```python
from build123d import *

# Parameters (mm, degrees)
BOSS_EXTRUDE1_DEPTH = 12.7
SKETCH2_R           = 2.286
SKETCH2_R_2         = 0.6
CUT_EXTRUDE1_DEPTH  = 3.175
FILLET1_R           = 2.54


with BuildPart() as part:
    # Sketch1 → Boss-Extrude1 (new body)
    with BuildSketch(Plane.XY):
        with BuildLine():
            Line((0, 26.364540169), (0, -11.735459831))
            ThreePointArc((0, -11.735459831), (0.371974388, -12.633485443), (1.27, -13.005459831))
            Line((1.27, -13.005459831), (13.97, -13.005459831))
            Line((13.97, -13.005459831), (13.97, -16.180459831))
            Line((13.97, -16.180459831), (1.27, -16.180459831))
            ThreePointArc((1.27, -16.180459831), (-1.873089642, -14.878549473), (-3.175, -11.735459831))
            Line((-3.175, -11.735459831), (-3.175, 26.364540169))
            Line((-3.175, 26.364540169), (0, 26.364540169))
        make_face()
    extrude(amount=BOSS_EXTRUDE1_DEPTH)

    # Sketch2 → Cut-Extrude1 (cut)
    with BuildSketch(Plane.ZY.offset(3.175)):
        with Locations(Location((6.35, 22.554540169, 0), (0, 0, 270))):
            Circle(SKETCH2_R)
        with Locations(Location((6.35, 8.104540169, 0), (0, 0, 270))):
            Circle(SKETCH2_R_2)
        with Locations(Location((6.35, 12.104540169, 0), (0, 0, 270))):
            Circle(SKETCH2_R_2)
        with Locations(Location((6.35, 16.104540169, 0), (0, 0, 270))):
            Circle(SKETCH2_R_2)
    extrude(amount=-CUT_EXTRUDE1_DEPTH, mode=Mode.SUBTRACT)

    # Fillet1
    fillet1_edges = [part.edges().sort_by_distance(p)[0] for p in [
        (-1.5875, 26.364540169, 0),
        (13.97, -14.592959831, 12.7),
        (-1.5875, 26.364540169, 12.7),
        (13.97, -14.592959831, 0),
    ]]
    fillet(fillet1_edges, radius=FILLET1_R)


solid = part.part
```
Geometry check sheet. Reference: the model listing, model coordinates, mm. A direction names the side the tool comes from. Round coordinates to 2 decimals unless told otherwise and drop trailing zeros. Order: outer loops, then holes, each group sorted by start corner. A loop starts at its lowest first (then second) coordinate and runs counter-clockwise, first axis right, second up. Notation, with made-up numbers: (34, 86) - (91, 86) arc R31 cw to (91, 113) - close; hole circle Ø5 at (-39.5, 48.5). An arc over 180 degrees is marked (long way). Use a Markdown table: item, result. Add a question column.
(1) Depth check by flat-ended pin: pin 1 (1.9 mm diameter, centred on y = 8.1, z = 6.35, fed in from +X); pin 2 (6.5 mm diameter, centred on x = 7, z = 8, fed in from +Y); pin 3 (8 mm diameter, centred on x = 11.5, y = -6.5, fed in from +Z). Enter the tip coordinate at first touch or a pass-through.
(2) Tool access check on faces 1 (the flat face through (-2, 26.365, 6)), 2 (the flat face through (8, -13.005, 6)). Record the directions out of +Z, -Z, +X, -X, +Y, -Y that give a thin tool (end or side, any length) a straight path to the whole face; none if there is none.
(3) Material ranges on line 1 along Y through (x, z) = (5.75, 6.75); line 2 along X through (y, z) = (20, 3.25) (3 decimals); line 3 along Z through (x, y) = (-1.75, 23), recorded low to high. Write a range as [from, to].
(4) Sectioned sample at A-A, the plane z = 6.35. Enter the section's corners in (x, y) (3 decimals).
(5) Sectioned sample at B-B, the plane z = 9.5. Enter the section's corners in (x, y) (3 decimals), and give its area (3 significant figures).
(6) Sectioned sample at C-C, the plane x = -1.25. Enter the section's corners in (y, z), and give its area (3 significant figures).
(7) Release check for a two-part mould opening along Y. For faces 3 (the cylindrical face through (-1.61, 11.55, 6.12)), 4 (the flat face through (8, -16.18, 6)), 5 (the flat face through (13.97, -15, 6)) record: pulls with the +Y half, pulls with the -Y half, needs draft (parallel to the pull), parting line crosses it, or undercut.
(8) Sectioned sample at D-D, the plane y = -1. Enter the section's corners in (x, z) (3 decimals).
Answers below:
| question | item | result |
|---|---|---|
| 1 | pin 1 | x = 0 |
| 1 | pin 2 | y = -13.01 |
| 1 | pin 3 | through |
| 2 | face 1 | +Z, -Z, +X, -X, +Y |
| 2 | face 2 | +Z, -Z, +X, +Y |
| 3 | line 1 | [-16.18, -13.01] |
| 3 | line 2 | [-3.175, 0] |
| 3 | line 3 | [0, 4.11], [8.59, 12.7] |
| 4 | outline | (-3.175, -11.735) arc R4.445 ccw to (1.27, -16.18) - (13.97, -16.18) - (13.97, -13.005) - (1.27, -13.005) arc R1.27 cw to (0, -11.735) - (0, 7.505) - (-3.175, 7.505) - close; (-3.175, 8.705) - (0, 8.705) - (0, 11.505) - (-3.175, 11.505) - close; (-3.175, 12.705) - (0, 12.705) - (0, 15.505) - (-3.175, 15.505) - close; (-3.175, 16.705) - (0, 16.705) - (0, 20.269) - (-3.175, 20.269) - close; (-3.175, 24.841) - (0, 24.841) - (0, 26.365) - (-3.175, 26.365) - close |
| 5 | outline | (-3.175, -11.735) arc R4.445 ccw to (1.27, -16.18) - (13.97, -16.18) - (13.97, -13.005) - (1.27, -13.005) arc R1.27 cw to (0, -11.735) - (0, 26.365) - (-3.175, 26.365) - close |
| 5 | area | 176 mm² |
| 6 | outline | (-15.4, 0) - (23.82, 0) arc R2.54 ccw to (26.36, 2.54) - (26.36, 10.16) arc R2.54 ccw to (23.82, 12.7) - (-15.4, 12.7) - close; hole circle Ø1.2 at (8.1, 6.35); hole circle Ø1.2 at (12.1, 6.35); hole circle Ø1.2 at (16.1, 6.35); hole circle Ø4.57 at (22.55, 6.35) |
| 6 | area | 508 mm² |
| 7 | face 3 | undercut |
| 7 | face 4 | pulls with the -Y half |
| 7 | face 5 | needs draft |
| 8 | outline | (-3.175, 0) - (0, 0) - (0, 12.7) - (-3.175, 12.7) - close |
